Geometry: final body of the model. Coordinates: model frame, mm. A direction names the side the tool comes from. Give positions to 0.01 mm unless a question says otherwise; leave off trailing zeros. Write each loop counter-clockwise with the first axis right and the second up, starting at its lowest first coordinate (ties: lowest second). Pieces come first, ordered by that corner, then holes.
from build123d import *

# Parameters (mm, degrees)
SKETCH002_R  = 1.993559
POCKET_DEPTH = 0.5
FILLET_R     = 0.5


with BuildPart() as part:
    # Sketch → Revolution (revolve)
    with BuildSketch(Plane.XZ):
        with BuildLine():
            ThreePointArc((3.985235, 0), (2.344302, 1.802426), (0, 2.47))
            Line((0, 7.993666), (0, 2.47))
            Line((3.4821, 7.993666), (0, 7.993666))
            Line((3.4821, 7.008655), (3.4821, 7.993666))
            Line((2.5, 7.008655), (3.4821, 7.008655))
            Line((2.5, 5.015182), (2.5, 7.008655))
            Line((3.4821, 5.015182), (2.5, 5.015182))
            Line((3.4821, 3.959811), (3.4821, 5.015182))
            Line((2.050408, 3.959811), (3.4821, 3.959811))
            Line((2.050408, 3.075381), (2.050408, 3.959811))
            ThreePointArc((4.536749, 0), (3.55737, 1.750957), (2.050408, 3.075381))
            Line((3.985235, 0), (4.536749, 0))
        make_face()
    revolve(axis=Axis((0, 0, 0), (0, 0, 1)))

    # Sketch001 → Groove (revolve, cut)
    with BuildSketch(Plane.XZ):
        Polygon((1, 8.108983), (1, 4.197927), (1.533167, 2.20812), (0, 2.398983), (0, 8.108983), align=None)
    revolve(axis=Axis((0, 0, 0), (0, 0, 1)), mode=Mode.SUBTRACT)

    # Sketch002 (on Face8 of Groove) → Pocket (cut)
    with BuildSketch(Plane(origin=(0, 0, 7.993666), x_dir=(-1, 0, 0), z_dir=(0, 0, 1))):
        Circle(SKETCH002_R)
    extrude(amount=-POCKET_DEPTH, mode=Mode.SUBTRACT)

    # Fillet
    fillet_edges = [part.edges().sort_by_distance(p)[0] for p in [
        (-3.4821, 0, 7.993666),
    ]]
    fillet(fillet_edges, radius=FILLET_R)


solid = part.part
Q1. Access query for faces 1 (the flat face through (1, -2, 7.994)), 2 (the flat face through (0, -2.3, 3.96)), 3 (the cylindrical face through (-2.76, -2.12, 4.49)). Directions: +Z, -Z, +X, -X, +Y, -Y. A direction counts if a zero-diameter tool reaches every point of the face in a straight line with its end or side. Return the directions, or none.
Filled sheet:
face 1: +Z, +X, -X, +Y, -Y
face 2: none
face 3: +Z
Q2. Section A-A on z = 5.25. Output: boundary loops of the cut face in (x, y), plus the area to 3 significant figures.
Filled sheet:
outline: circle Ø5 at (0, 0); hole circle Ø2 at (0, 0)
area: 16.5 mm2
Q3. Pull-direction query (Y, two-part tool) for faces 4 (the cylindrical face through (0, -1, 6)), 5 (the cylindrical face through (-2.76, -2.12, 7.25)), 6 (the flat face through (-3, -3, 0)); classes: released by +Y, released by -Y, zero draft, split by the parting line, or undercut.
Filled sheet:
face 4: undercut
face 5: split by the parting line
face 6: zero draft
Q4. Pin query (flat end, axial travel): P1, Ø2, axis at y = 1.5, z = 4.5, coming from the -X side; P2, Ø1.5, axis at y = 1, z = 5, coming from the -X side; P3, Ø2, axis at y = -1, z = 1.5, coming from the -X side; P4, Ø1.5, axis at x = 0, y = -3.5, coming from the -Z side. Return the tip coordinate at first contact, or that it passes through.
Filled sheet:
P1: stops at x = -3.45
P2: stops at x = -3.47
P3: stops at x = -4.26
P4: stops at z = 0
Q5. Section B-B on z = 3.75. Output: boundary loops of the cut face in (x, y), plus the area to 3 significant figures.
Filled sheet:
outline: circle Ø4.1 at (0, 0); hole circle Ø2.24 at (0, 0)
area: 9.27 mm2
Q6. Ray query, line 1 along Y through (x, z) = (0, 6.35); line 2 along Z through (x, y) = (1, -2.5); line 3 along Y through (x, z) = (0, 4.9). Return the intervals inside material, ascending.
Filled sheet:
line 1: y = -2.5 to -1, 1 to 2.5
line 2: z = 1.56 to 2.62, 3.96 to 5.02, 7.01 to 7.99
line 3: y = -3.48 to -1, 1 to 3.48
